```python
from build123d import *

# Parameters (mm, degrees)
F1_DEPTH = 104.14
F2_W     = 101.6
F2_H     = 50.960924
F3_DEPTH = 25.4


with BuildPart() as f1:
    # F0 (on Right) → F1 (new body, symmetric)
    with BuildSketch(Plane.YZ):
        Polygon((-101.6, 0), (0, 0), (0, 88.9), (-31.75, 88.9), (-44.45, 31.75), (-101.6, 31.75), align=None)
    extrude(amount=F1_DEPTH, both=True)

    # F2 (on face) → F3 (join)
    with BuildSketch(Plane.YZ.offset(104.14)):
        with Locations((-50.8, 25.480462)):
            Rectangle(F2_W, F2_H)
    extrude(amount=-F3_DEPTH)

    # F4: F1 across plane


with BuildPart() as f1_1:
    add(f1.part)
    add(f1.part.mirror(Plane.YZ))


solid = f1_1.part
```
Here's how the part is built. I have some questions about the finished solid (model axes, mm). A direction names the side the tool comes from. Round coordinates to 2 decimals unless told otherwise and drop trailing zeros. Loops run counter-clockwise (first coordinate to the right, second up) from the corner with the lowest first, then second, coordinate; pieces in that order, holes last. Notation, with made-up numbers: (49.25, 36) -> (92.25, 36) arc R24 cw to (92.25, 73) -> close; hole circle Ø3 at (-17.5, 49.5). An arc over 180 degrees is marked (long way). Answer as CSV lines item,"result". Start each with the question number.
1. Imagine slicing it at B-B on y = -59. Write out the boundary of the cut face in (x, z), plus the area to 3 significant figures.
2. Imagine slicing it at A-A on z = 43. Write out the boundary of the cut face in (x, y), plus the area to 3 significant figures.
3. For faces 1 (the face through (78.74, -71, 41)), 2 (the face through (1, -101.6, 20)), 3 (the face through (92, -71, 50.961)), which set-ups out of +Z, -Z, +X, -X, +Y, -Y let a thin tool reach every point of the face, with its end or its side?
4. I need wall thicknesses on probe 1 along X at (y, z) = (-69.5, 34); probe 2 along Z at (x, y) = (-29, -46); probe 3 along Z at (x, y) = (-88, -94). Which ranges of each line are inside material? Lowest first, please. Write a range as from..to.
5. Imagine slicing it at C-C on x = -41.5. Write out the boundary of the cut face in (y, z), plus the area to 3 significant figures.
6. If we mould it in two halves opening along X, with no side actions, what happens to faces 4 (the face through (1, -73, 31.75)), 5 (the face through (-104.14, -40, 35)), 6 (the face through (1, -16, 88.9))? For each: pulls with the +X half, pulls with the -X half, needs draft (parallel to the pull), parting line crosses it, or undercut.
7. Imagine slicing it at D-D on z = 73.5. Write out the boundary of the cut face in (x, y), plus the area to 3 significant figures.
8. I'm going to push flat-ended pins straight in: P1, Ø7.5, axis at x = -95, y = -75, coming from the +Z side; P2, Ø12, axis at x = -11.5, y = -72.5, coming from the +Z side. Where does each tip first touch, or does it pass through?
Solution:
1,outline,"(-104.14, 0) -> (104.14, 0) -> (104.14, 50.96) -> (78.74, 50.96) -> (78.74, 31.75) -> (-78.74, 31.75) -> (-78.74, 50.96) -> (-104.14, 50.96) -> close"
1,area,"7,590 mm²"
2,outline,"(-104.14, -101.6) -> (-78.74, -101.6) -> (-78.74, -41.95) -> (78.74, -41.95) -> (78.74, -101.6) -> (104.14, -101.6) -> (104.14, 0) -> (-104.14, 0) -> close"
2,area,"11,800 mm²"
3,face 1,"+Z, -Y"
3,face 2,"+Z, -Z, +X, -X, -Y"
3,face 3,"+Z, +X, -X, -Y"
4,probe 1,"-104.14..-78.74, 78.74..104.14"
4,probe 2,"0..31.75"
4,probe 3,"0..50.96"
5,outline,"(-101.6, 0) -> (0, 0) -> (0, 88.9) -> (-31.75, 88.9) -> (-44.45, 31.75) -> (-101.6, 31.75) -> close"
5,area,"5,400 mm²"
6,face 4,"undercut"
6,face 5,"pulls with the -X half"
6,face 6,"needs draft"
7,outline,"(-104.14, -35.17) -> (104.14, -35.17) -> (104.14, 0) -> (-104.14, 0) -> close"
7,area,"7,330 mm²"
8,P1,"z = 50.96"
8,P2,"z = 31.75"
